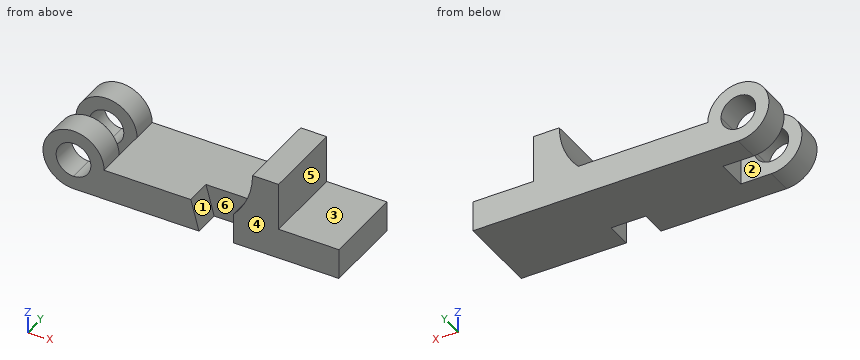
```python
from build123d import *

# Parameters (mm, degrees)
F0_W     = 19.05
F0_H     = 34.798
F1_DEPTH = 30.1625
F3_DEPTH = 19.05
F5_W     = 44.704
F5_H     = 22.3266
F6_DEPTH = 49.531


with BuildPart() as f1:
    # F0 (on Front) → F1 (new body, symmetric)
    with BuildSketch(Plane.XZ):
        Polygon((97.1042, 0), (97.1042, 22.352), (52.9844, 22.352), (33.9344, 22.352), (20.1443877871, 22.352), (20.1443877871, 0), align=None)
        with Locations((43.4594, 39.751)):
            Rectangle(F0_W, F0_H)
        with BuildLine():
            Line((20.1443877871, 22.352), (33.9344, 22.352))
            Line((33.9344, 22.352), (33.9344, 57.15))
            ThreePointArc((33.9344, 57.15), (30.3612323074, 38.4345969798), (20.1443877871, 22.352))
        make_face()
        with BuildLine():
            Line((-97.1042, 0), (20.1443877871, 0))
            Line((20.1443877871, 0), (20.1443877871, 22.352))
            Line((20.1443877871, 22.352), (-74.7522, 22.352))
            ThreePointArc((-74.7522, 22.352), (-81.2989492269, 6.5467492269), (-97.1042, 0))
        make_face()
        with BuildLine():
            ThreePointArc((-74.7522, 22.352), (-112.9094507731, 38.1572507731), (-97.1042, 0))
            Line((-97.1042, 0), (-97.1042, 9.652))
            ThreePointArc((-97.1042, 9.652), (-106.0844561211, 31.3322561211), (-84.4042, 22.352))
            Line((-84.4042, 22.352), (-74.7522, 22.352))
        make_face()
        with BuildLine():
            Line((-97.1042, 9.652), (-97.1042, 0))
            ThreePointArc((-97.1042, 0), (-81.2989492269, 6.5467492269), (-74.7522, 22.352))
            Line((-74.7522, 22.352), (-84.4042, 22.352))
            ThreePointArc((-84.4042, 22.352), (-88.1239438789, 13.3717438789), (-97.1042, 9.652))
        make_face()
    extrude(amount=F1_DEPTH, both=True)

    # F2 (on face) → F3 (cut)
    with BuildSketch(Plane.XZ.offset(30.1625)):
        Polygon((-5.2578, 0), (20.1443877871, 0), (20.1443877871, 22.352), (-11.2522, 22.352), align=None)
    extrude(amount=-F3_DEPTH, mode=Mode.SUBTRACT)

    # F5 (on offset) → F6 (cut, through all)
    with BuildSketch(Plane.XY.offset(49.53)):
        with Locations((-97.1042, 0)):
            Rectangle(F5_W, F5_H)
    extrude(amount=-F6_DEPTH, mode=Mode.SUBTRACT)


solid = f1.part
```
Input: part model. Units: mm. Frame: model coordinates. Face numbers are marked on the shaded views. A direction names the side the tool comes from. Give positions to 0.01 mm unless a question says otherwise; leave off trailing zeros. Write each loop counter-clockwise with the first axis right and the second up, starting at its lowest first coordinate (ties: lowest second). Pieces come first, ordered by that corner, then holes. Notation, with made-up numbers: (59, 36) - (82, 36) arc R20 cw to (82, 46) - close; hole circle Ø7 at (19, 61). An arc over 180 degrees is marked (long way). Write item = value, one per line. Start each with the question number.
1. First-contact query: pin 1 Ø10 at (y, z) = (8.5, 14) entering from -X; pin 2 Ø8 at (y, z) = (14, 46.5) entering from +X; pin 3 Ø24.5 at (x, z) = (7.5, 14.5) entering from -Y; pin 4 Ø23 at (x, z) = (-97.1, 22.35) entering from -Y. Flat tips, straight axial feed; report the tip coordinate or a pass-through.
2. Access query for the marked faces 1, 2 and 3. Directions: +Z, -Z, +X, -X, +Y, -Y. A direction counts if a zero-diameter tool reaches every point of the face in a straight line with its end or side. Return the directions, or none.
3. Section query A-A, the plane z = 41. Output: boundary loops of the cut face in (x, y).
4. Section query C-C, the plane x = -81. Output: boundary loops of the cut face in (y, z).
5. Section query D-D, the plane z = 30. Output: boundary loops of the cut face in (x, y).
6. Section query B-B, the plane y = 20.5. Output: boundary loops of the cut face in (x, z), then the cut area to 3 significant figures.
7. Ray query, L1, parallel to X at y = -21.5, z = 23; L2, parallel to Y at x = -77, z = 30; L3, parallel to X at y = -13, z = 14.5. Return the intervals inside material, ascending.
8. Mould query, pull axis X, two halves, no side actions, for the marked faces 4, 5 and 6. Classes: released by +X, released by -X, zero draft, split by the parting line, or undercut.
Check sheet entries:
q1.pin_1 = -119.07
q1.pin_2 = 52.98
q1.pin_3 = -11.11
q1.pin_4 = through
q2.face_1 = +Z, -Y
q2.face_2 = +Z, -Z, -X
q2.face_3 = +Z, +X, +Y, -Y
q3.outline = (-109.43, -30.16) - (-84.78, -30.16) - (-84.78, -11.16) - (-109.43, -11.16) - close; (-109.43, 11.16) - (-84.78, 11.16) - (-84.78, 30.16) - (-109.43, 30.16) - close; (31.3, -30.16) - (52.98, -30.16) - (52.98, 30.16) - (31.3, 30.16) - close
q4.outline = (-30.16, 0) - (-11.16, 0) - (-11.16, 37.85) - (-30.16, 37.85) - close; (11.16, 0) - (30.16, 0) - (30.16, 37.85) - (11.16, 37.85) - close
q5.outline = (-118.11, -30.16) - (-107.24, -30.16) - (-107.24, -11.16) - (-118.11, -11.16) - close; (-118.11, 11.16) - (-107.24, 11.16) - (-107.24, 30.16) - (-118.11, 30.16) - close; (-86.97, -30.16) - (-76.1, -30.16) - (-76.1, -11.16) - (-86.97, -11.16) - close; (-86.97, 11.16) - (-76.1, 11.16) - (-76.1, 30.16) - (-86.97, 30.16) - close; (26.07, -30.16) - (52.98, -30.16) - (52.98, 30.16) - (26.07, 30.16) - close
q6.outline = (-97.1, 0) - (97.1, 0) - (97.1, 22.35) - (52.98, 22.35) - (52.98, 57.15) - (33.93, 57.15) arc R50.8 cw to (20.14, 22.35) - (-74.75, 22.35) arc R22.35 ccw (long way) to start; hole circle Ø25.4 at (-97.1, 22.35)
q6.area = 5,820 mm2
q7.L1 = -119.45 to -109.79, -84.42 to -74.76, 20.74 to 52.98
q7.L2 = -30.16 to -11.16, 11.16 to 30.16
q7.L3 = -118.03 to -107.09, -87.12 to -9.15, 20.14 to 97.1
q8.face_4 = zero draft
q8.face_5 = released by +X
q8.face_6 = undercut
